Design review of the part built by this model. Coordinates are the model's own, in mm. Face numbers are marked on the shaded views. A direction names the side the tool comes from. Coordinates: 2 decimals unless noted, no trailing zeros. Write each loop counter-clockwise with the first axis right and the second up, starting at its lowest first coordinate (ties: lowest second). Pieces come first, ordered by that corner, then holes.
Q1. For probe 1 along Y at (x, z) = (-37.5, 44.25); probe 2 along X at (y, z) = (-3.75, 40.25); probe 3 along Z at (x, y) = (-53.5, -9.75), list the stretches that pass through material, from the lowest coordinate up.
Q2. Insertion check: pin 1 (4.5 mm diameter, centred on x = -54, y = -6, fed in from -Z); pin 2 (3 mm diameter, centred on x = -47.5, y = -7.5, fed in from +Z); pin 3 (6 mm diameter, centred on y = -5, z = 34.5, fed in from +X). Each pin has a flat end and moves straight along its axis. Give the tip position at first contact, or say it passes through.
Q3. Mouldability with a two-part tool opening along Y and no side actions: class the marked faces 1, 2 and 3 as pulls with the +Y half, pulls with the -Y half, needs draft (parallel to the pull), parting line crosses it, or undercut.
Q4. Take a section at B-B (z = 26). Give the boundary of the cut face in (x, y), and give its area (3 significant figures).
Q5. Take a section at C-C (y = -10.5). Give the boundary of the cut face in (x, z), and give its area (3 significant figures).
Q6. Take a section at A-A (x = -57). Give the boundary of the cut face in (y, z).
Q7. Machinability: for the marked faces 4, 5 and 6, which of the approach directions +Z, -Z, +X, -X, +Y, -Y give a long, thin tool a straight path to every point of the face, cutting with its end or side? Answer none if there is none.
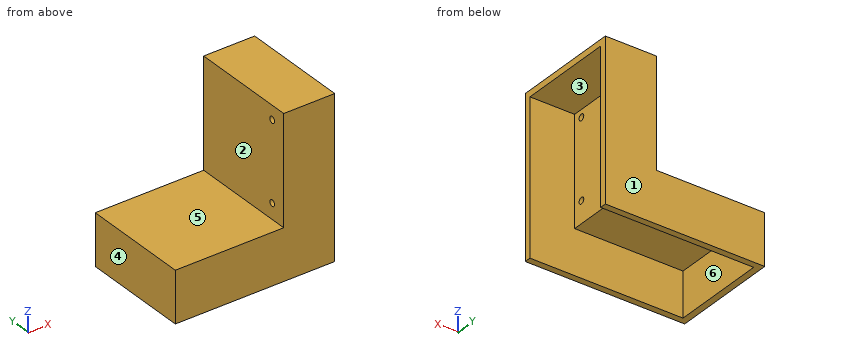
```python
from build123d import *

# Parameters (mm, degrees)
F0_W     = 17
F0_H     = 8
F0_W_2   = 8
F0_H_2   = 17
F1_DEPTH = 17
F2_W     = 24
F2_H     = 15
F3_DEPTH = 7
F4_W     = 15
F4_H     = 17
F5_DEPTH = 7
F7_D     = 1


with BuildPart() as f1:
    # F0 (on Front) → F1 (new body)
    with BuildSketch(Plane.XZ):
        with Locations((-51.656717, 24.650854)):
            Rectangle(F0_W, F0_H)
        with Locations((-39.156717, 37.150854)):
            Rectangle(F0_W_2, F0_H_2)
        with Locations((-39.156717, 24.650854)):
            Rectangle(F0_W_2, F0_H)
    extrude(amount=F1_DEPTH)

    # F2 (on face) → F3 (cut)
    with BuildSketch(Plane(origin=(0, 0, 20.650854), x_dir=(1, 0, 0), z_dir=(0, 0, -1))):
        with Locations((-47.156717, 8.5)):
            Rectangle(F2_W, F2_H)
    extrude(amount=-F3_DEPTH, mode=Mode.SUBTRACT)

    # F4 (on face) → F5 (cut)
    with BuildSketch(Plane.YZ.offset(-35.156717)):
        with Locations((-8.5, 36.150854)):
            Rectangle(F4_W, F4_H)
    extrude(amount=-F5_DEPTH, mode=Mode.SUBTRACT)

    # F7 (through all)
    with Locations(Plane.YZ.offset(-42.156717)):
        with Locations((-14.552529, 31.091157), (-14.552529, 43.474194)):
            Hole(F7_D / 2)


solid = f1.part
```
Response:
1. probe 1: y = -17 to -16, -1 to 0
1. probe 2: x = -43.16 to -42.16
1. probe 3: z = 27.65 to 28.65
2. pin 1: stops at z = 27.65
2. pin 2: stops at z = 28.65
2. pin 3: stops at x = -42.16
3. face 1: pulls with the +Y half
3. face 2: needs draft
3. face 3: undercut
4. outline: (-60.16, -17) - (-35.16, -17) - (-35.16, -16) - (-59.16, -16) - (-59.16, -1) - (-35.16, -1) - (-35.16, 0) - (-60.16, 0) - close
4. area: 65.0 mm2
5. outline: (-60.16, 20.65) - (-59.16, 20.65) - (-59.16, 27.65) - (-42.16, 27.65) - (-42.16, 44.65) - (-35.16, 44.65) - (-35.16, 45.65) - (-43.16, 45.65) - (-43.16, 28.65) - (-60.16, 28.65) - close
5. area: 49.0 mm2
6. outline: (-17, 20.65) - (-16, 20.65) - (-16, 27.65) - (-1, 27.65) - (-1, 20.65) - (0, 20.65) - (0, 28.65) - (-17, 28.65) - close
7. face 4: +Z, -Z, -X, +Y, -Y
7. face 5: +Z, -X, +Y, -Y
7. face 6: -Z, +X
